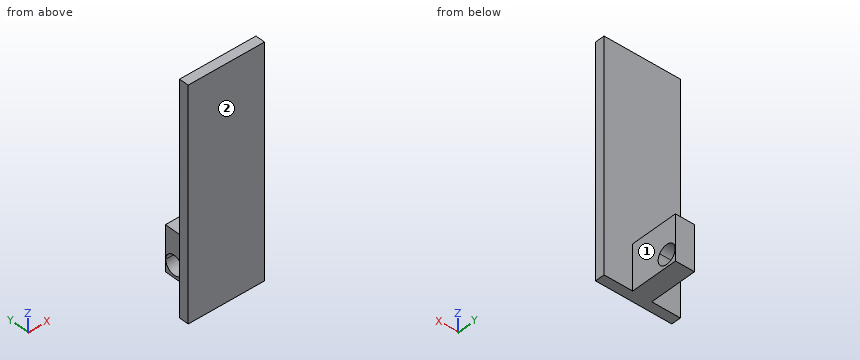
from build123d import *

# Parameters (mm, degrees)
F0_W     = 50.8
F0_H     = 152.4
F1_DEPTH = 6.35
F2_W     = 12.7
F2_H     = 30.0863
F3_DEPTH = 31.75
F6_DEPTH = 31.751


with BuildPart() as f1:
    # F0 (on Front) → F1 (new body)
    with BuildSketch(Plane.XZ):
        Rectangle(F0_W, F0_H)
    extrude(amount=F1_DEPTH)

    # F2 (on face) → F3 (join)
    with BuildSketch(Plane(origin=(0, 0, 0), x_dir=(-1, 0, 0), z_dir=(0, 1, 0))):
        with Locations((0, -61.15685)):
            Rectangle(F2_W, F2_H)
    extrude(amount=F3_DEPTH)

    # F5 (on face) → F6 (cut, through all)
    with BuildSketch(Plane.YZ.offset(6.35)):
        with BuildLine():
            ThreePointArc((20.0271333182, -64.5413445885), (25.26483083, -67.5054111988), (30.6239423072, -64.7669645094))
            ThreePointArc((30.6239423072, -64.7669645094), (25.3862447954, -61.802897899), (20.0271333182, -64.5413445885))
        make_face()
        with BuildLine():
            ThreePointArc((20.0271333182, -64.5413445885), (23.3602469249, -74.2134114917), (31.6010756254, -68.1514590979))
            ThreePointArc((31.6010756254, -68.1514590979), (31.3519035786, -66.3900964761), (30.6239423072, -64.7669645094))
            ThreePointArc((30.6239423072, -64.7669645094), (25.26483083, -67.5054111988), (20.0271333182, -64.5413445885))
        make_face()
    extrude(amount=-F6_DEPTH, mode=Mode.SUBTRACT)


solid = f1.part
Verification items for the finished model (mm, model axes). Face numbers are marked on the shaded views. A direction names the side the tool comes from. Give positions to 0.01 mm unless a question says otherwise; leave off trailing zeros. Order: outer loops, then holes, each group sorted by start corner. A loop starts at its lowest first (then second) coordinate and runs counter-clockwise, first axis right, second up. Notation, with made-up numbers: M 89.5,57 L 126.5,57 A20 cw 126.5,68 Z; hole C 23,43 d5. An arc over 180 degrees is marked long. Answer as a JSON object with one key per item and string values. Group by question number.
1) Depth check by flat-ended pin: pin 1 Ø15 at (x, z) = (-8, -10.5) entering from +Y; pin 2 Ø14 at (x, y) = (0, 11) entering from +Z; pin 3 Ø5 at (y, z) = (10.5, -53.5) entering from -X; pin 4 Ø8 at (y, z) = (4.5, 27) entering from +X. Enter the tip coordinate at first touch or a pass-through.
2) Scan lines: line 1 along Y through (x, z) = (23.5, 38); line 2 along X through (y, z) = (3, -47). Record each from-to range of solid material in increasing order. Write a range as [from, to].
3) Cross-section at A-A (x = -1). Enter the section's corners in (y, z).
4) Cross-section at D-D (x = 16). Enter the section's corners in (y, z), then the cut area to 3 significant figures.
5) Cross-section at C-C (y = 25.5). Enter the section's corners in (x, z), then the cut area to 3 significant figures.
6) Cross-section at B-B (z = -57). Enter the section's corners in (x, y), then the cut area to 3 significant figures.
7) Access from +Z, -Z, +X, -X, +Y, -Y to the whole of each face (thin tool, end or side, straight path). Record for the marked faces 1 and 2.
Result sheet:
{
 "1": {"pin 1": "stops at y = 0", "pin 2": "stops at z = -46.11", "pin 3": "stops at x = -6.35", "pin 4": "passes through"},
 "2": {"line 1": "y = [-6.35, 0]", "line 2": "x = [-6.35, 6.35]"},
 "3": {"outline": "M -6.35,-76.2 L 31.75,-76.2 L 31.75,-46.11 L 0,-46.11 L 0,76.2 L -6.35,76.2 Z; hole C 25.25,-68.15 d12.7"},
 "4": {"outline": "M -6.35,-76.2 L 0,-76.2 L 0,76.2 L -6.35,76.2 Z", "area": "968 mm2"},
 "5": {"outline": "M -6.35,-76.2 L 6.35,-76.2 L 6.35,-74.5 L -6.35,-74.5 Z; M -6.35,-61.81 L 6.35,-61.81 L 6.35,-46.11 L -6.35,-46.11 Z", "area": "221 mm2"},
 "6": {"outline": "M -25.4,-6.35 L 25.4,-6.35 L 25.4,0 L 6.35,0 L 6.35,31.75 L -6.35,31.75 L -6.35,0 L -25.4,0 Z", "area": "726 mm2"},
 "7": {"face 1": "+Z, -Z, +X, +Y", "face 2": "+Z, -Z, +X, -X, -Y"}
}
